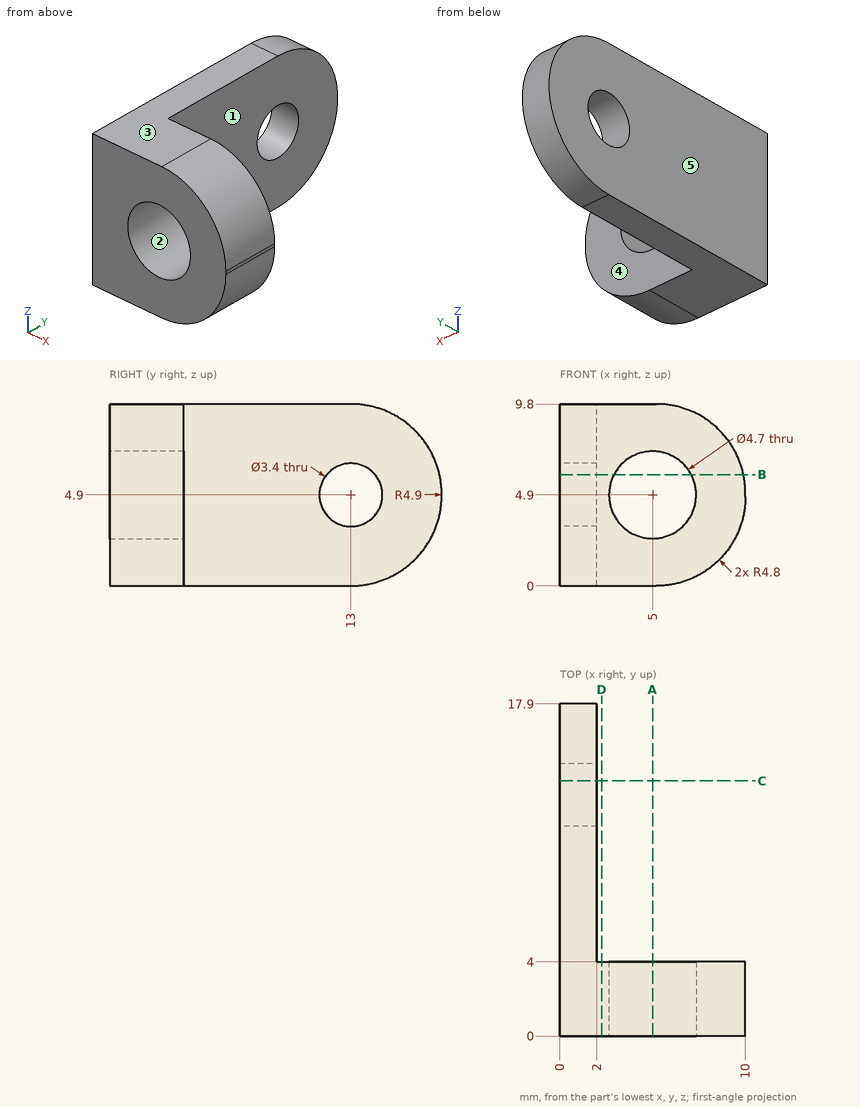
For this review, use the dimensioned drawing (mm, ordinates from the lowest corner) and the shaded views. A direction names the side the tool comes from. Coordinates: 2 decimals unless noted, no trailing zeros. Write each loop counter-clockwise with the first axis right and the second up, starting at its lowest first coordinate (ties: lowest second). Pieces come first, ordered by that corner, then holes. Notation, with made-up numbers: (-16, 8.25) -> (19, 8.25) arc R5 ccw to (19, 16.25) -> close; hole circle Ø9 at (-4.5, -26.75). An arc over 180 degrees is marked (long way). Put each result on its own line as item: value.
Q1. Take a section at A-A, the plane x = 5. State the section outline as (y, z) points.
From the geometry:
outline: (0, 0) -> (4, 0) -> (4, 2.55) -> (0, 2.55) -> close; (0, 7.25) -> (4, 7.25) -> (4, 9.8) -> (0, 9.8) -> close
Q2. The part is to be moulded in two halves that separate along Z. For the marked faces 1, 2 and 3, say which applies: +Z half, -Z half, draft (parallel to the pull), parting line (faces both ways), or undercut.
From the geometry:
face 1: draft
face 2: undercut
face 3: +Z half
Q3. Take a section at C-C, the plane y = 13.75. State the section outline as (x, z) points.
From the geometry:
outline: (0, 0.06) -> (2, 0.06) -> (2, 3.37) -> (0, 3.37) -> close; (0, 6.43) -> (2, 6.43) -> (2, 9.74) -> (0, 9.74) -> close
Q4. Take a section at D-D, the plane x = 2.25. State the section outline as (y, z) points, then the cut area to 3 significant figures.
From the geometry:
outline: (0, 0) -> (4, 0) -> (4, 9.8) -> (0, 9.8) -> close
area: 39.2 mm2
Q5. Take a section at B-B, the plane z = 6. State the section outline as (x, y) points.
From the geometry:
outline: (0, 0) -> (2.92, 0) -> (2.92, 4) -> (2, 4) -> (2, 11.7) -> (0, 11.7) -> close; (0, 14.3) -> (2, 14.3) -> (2, 17.77) -> (0, 17.77) -> close; (7.08, 0) -> (9.89, 0) -> (9.89, 4) -> (7.08, 4) -> close
Q6. Clearance check with flat-ended pins moving along their axes: pin 1 Ø4 at (x, z) = (4.5, 2.5) entering from +Y; pin 2 Ø4.5 at (y, z) = (13, 4.9) entering from +X; pin 3 Ø3 at (x, y) = (3, 14.5) entering from -Z; pin 4 Ø4 at (x, z) = (5, 4.9) entering from -Y. State where each tip first meets the part, or that it passes through.
From the geometry:
pin 1: stops at y = 4
pin 2: stops at x = 2
pin 3: stops at z = 0.01
pin 4: passes through
Q7. Tool access review of the marked faces 4 and 5: name each direction out of +Z, -Z, +X, -X, +Y, -Y from which nothing blocks a thin tool from reaching the whole face with its end or side.
From the geometry:
face 4: +Z, -Z, +X, +Y
face 5: +Z, -Z, -X, +Y, -Y
Q8. Wall thickness on L1, parallel to Z at x = 1.5, y = 13; L2, parallel to X at y = 2.45, z = 4.9; L3, parallel to X at y = 16, z = 2.75: over which ranges is each line inside the solid? List them lowest first.
From the geometry:
L1: z = 0 to 3.2, 6.6 to 9.8
L2: x = 0 to 2.65, 7.35 to 10
L3: x = 0 to 2
